```python
from build123d import *

# Parameters (mm, degrees)
BOSS_EXTRUDE1_DEPTH = 6.35
SKETCH8_W           = 4.7625
SKETCH8_H           = 14.2875
SKETCH8_W_2         = 9.525
SKETCH8_H_2         = 3.175
CUT_EXTRUDE5_DEPTH  = 6.35
SKETCH9_W           = 5.842
SKETCH9_H           = 13.716
CUT_EXTRUDE6_DEPTH  = 6.35


with BuildPart() as part:
    # Sketch7 → Boss-Extrude1 (new body)
    with BuildSketch(Plane.XY):
        Polygon((6.35, -25.4), (12.7, -25.4), (12.7, 25.4), (-12.7, 25.4), (-12.7, -25.4), (-6.35, -25.4), (-6.35, -12.7), (6.35, -12.7), align=None)
    extrude(amount=BOSS_EXTRUDE1_DEPTH)

    # Sketch8 → Cut-Extrude5 (cut)
    with BuildSketch(Plane.XY.offset(6.35)):
        with Locations((0, -5.55625)):
            Rectangle(SKETCH8_W, SKETCH8_H)
        with Locations((0, -3.175)):
            Rectangle(SKETCH8_W_2, SKETCH8_H_2)
    extrude(amount=-CUT_EXTRUDE5_DEPTH, mode=Mode.SUBTRACT)

    # Sketch9 → Cut-Extrude6 (cut)
    with BuildSketch(Plane.XY.offset(6.35)):
        with Locations((0, 12.7)):
            Rectangle(SKETCH9_W, SKETCH9_H)
    extrude(amount=-CUT_EXTRUDE6_DEPTH, mode=Mode.SUBTRACT)


solid = part.part
```
Read the model definition and answer for the solid it produces. Units are mm, in the model's axes. A direction names the side the tool comes from. Round coordinates to 2 decimals unless told otherwise and drop trailing zeros. Write each loop counter-clockwise with the first axis right and the second up, starting at its lowest first coordinate (ties: lowest second). Pieces come first, ordered by that corner, then holes. Notation, with made-up numbers: M 76.5,40 L 95.5,40 A21 cw 95.5,79 Z; hole C 85,-22.75 d5. An arc over 180 degrees is marked long. One line per item, written item: value.
Q1. Flat-ended cylindrical pins translate along their axes: pin 1 Ø2.5 at (x, z) = (3, 3) entering from -Y; pin 2 Ø2.5 at (x, z) = (1, 3.5) entering from -Y. Find the tip coordinate at first contact, or state that the pin passes through.
Data:
pin 1: y = -12.7
pin 2: y = 1.59
Q2. Find section D-D on x = 5.5. Write down the section's boundary in (y, z).
Data:
outline: M -12.7,0 L 25.4,0 L 25.4,6.35 L -12.7,6.35 Z
Q3. Find section C-C on z = 3. Write down the section's boundary in (x, y), plus the area to 3 significant figures.
Data:
outline: M -12.7,-25.4 L -6.35,-25.4 L -6.35,-12.7 L -2.38,-12.7 L -2.38,-4.76 L -4.76,-4.76 L -4.76,-1.59 L -2.38,-1.59 L -2.38,1.59 L 2.38,1.59 L 2.38,-1.59 L 4.76,-1.59 L 4.76,-4.76 L 2.38,-4.76 L 2.38,-12.7 L 6.35,-12.7 L 6.35,-25.4 L 12.7,-25.4 L 12.7,25.4 L -12.7,25.4 Z; hole M -2.92,5.84 L 2.92,5.84 L 2.92,19.56 L -2.92,19.56 Z
area: 966 mm2
Q4. Straight lines are drawn through the part: line 1 (X direction, y = 19.5, z = 2.75); line 2 (Y direction, x = 4, z = 2); line 3 (X direction, y = -17, z = 4.5). For each, find the intervals that lie inside material, in ascending order. Write a range as [from, to].
Data:
line 1: [-12.7, -2.92], [2.92, 12.7]
line 2: [-12.7, -4.76], [-1.59, 25.4]
line 3: [-12.7, -6.35], [6.35, 12.7]
Q5. For a pull along X with two mould halves and no side action, classify faces 4 (the flat face through (-3, 0, 6.35)), 5 (the flat face through (0, 19.558, 3)), 6 (the flat face through (12.7, 0, 3)), 7 (the flat face through (-12.7, 0, 3)) as +X half, -X half, draft (parallel to the pull), parting line (faces both ways), or undercut.
Data:
face 4: draft
face 5: undercut
face 6: +X half
face 7: -X half
Q6. Find section B-B on y = 12. Write down the section's boundary in (x, z), plus the area to 3 significant figures.
Data:
outline: M -12.7,0 L -2.92,0 L -2.92,6.35 L -12.7,6.35 Z; M 2.92,0 L 12.7,0 L 12.7,6.35 L 2.92,6.35 Z
area: 124 mm2
Q7. Find section A-A on x = 0.5. Write down the section's boundary in (y, z), plus the area to 3 significant figures.
Data:
outline: M 1.59,0 L 5.84,0 L 5.84,6.35 L 1.59,6.35 Z; M 19.56,0 L 25.4,0 L 25.4,6.35 L 19.56,6.35 Z
area: 64.1 mm2
Q8. Which of the six approach directions +Z, -Z, +X, -X, +Y, -Y give full straight-line access (tool end or side, diameter ignored) to faces 1 (the flat face through (6.35, -19, 3)), 2 (the flat face through (-10, -25.4, 3)), 3 (the flat face through (4.762, -3, 3))?
Data:
face 1: +Z, -Z, -Y
face 2: +Z, -Z, +X, -X, -Y
face 3: +Z, -Z
